Autodesk Inventor part; units mm, degrees
ref_plane "YZ Plane" through (0, 0, 0) normal (1, 0, 0) x (0, 1, 0)
ref_plane "XZ Plane" through (0, 0, 0) normal (0, 1, 0) x (-1, 0, 0)
ref_plane "XY Plane" through (0, 0, 0) normal (0, 0, 1) x (1, 0, 0)
sketch "Sketch1" plane through (0, 0, 0) normal (0, 1, 0) x (-1, 0, 0)
  line L0 (12.7, 14.875) -> (-12.7, 14.875)
  line L1 (-12.7, 14.875) -> (-12.7, -14.875)
  line L2 (-12.7, -14.875) -> (12.7, -14.875)
  line L3 (12.7, -14.875) -> (12.7, 14.875)
  point P0 (0, 0)
  dimension "d0" = 29.75
  dimension "d1" = 25.4
  dimension "d2" = 12.7
  dimension "d3" = 14.875
extrude "Extrusion1" add sketch "Sketch1" along normal blind 29.8
sketch "Sketch2" plane through (0, 29.8, 0) normal (0, 1, 0) x (1, 0, 0)
  circle A0 centre (0, 0) radius 5.35
  line L0 (12.7, 14.875) -> (-12.7, 14.875)
  line L1 (-12.7, 14.875) -> (-12.7, -14.875)
  line L2 (-12.7, -14.875) -> (12.7, -14.875)
  dimension "d7" = 10.7
  dimension "d8" = 14.875
  dimension "d9" = 12.7
  dimension "d12" = 14.875
extrude "Extrusion2" cut sketch "Sketch2" against normal through all
sketch "Sketch3" plane through (-12.7, 0, 14.875) normal (0, 0, 1) x (1, 0, 0)
  circle A0 centre (4.9, 24.9) radius 1.9
  circle A1 centre (21.4, 24.9) radius 1.9
  circle A2 centre (20.5, 4.9) radius 1.9
  circle A3 centre (4.9, 4.9) radius 1.9
  line L0 (0, 29.8) -> (25.4, 29.8)
  line L1 (0, 0) -> (0, 29.8)
  line L2 (0, 0) -> (25.4, 0)
  line L3 (25.4, 0) -> (25.4, 29.8)
  point P0 (12.7, 0)
  dimension "d13" = 3.8
  dimension "d14" = 3.8
  dimension "d15" = 3.8
  dimension "d16" = 3.8
  dimension "d17" = 4.9
  dimension "d18" = 4.9
  dimension "d19" = 4.9
  dimension "d20" = 4.9
  dimension "d21" = 4.9
  dimension "d22" = 4.9
  dimension "d23" = 4.9
  dimension "d24" = 4
hole "Hole1" at (-7.8, 24.9, 14.875) at (8.7, 24.9, 14.875) at (7.8, 4.9, 14.875) at (-7.8, 4.9, 14.875) direction (0, 0, -1) diameter 3.242 depth 11 tip angle 118 countersink diameter 4.3 countersink angle 90
sketch "Sketch4" plane through (0, 0, 0) normal (0, -1, 0) x (1, 0, 0)
  circle A0 centre (8, 0) radius 1.5
  circle A1 centre (0, -8) radius 1.5
  circle A2 centre (-8, 0) radius 1.5
  circle A3 centre (0, 8) radius 1.5
  line L0 (12.7, 14.875) -> (12.7, -14.875)
  line L1 (-12.7, -14.875) -> (-12.7, 14.875)
  line L2 (-12.7, 14.875) -> (12.7, 14.875)
  line L3 (12.7, -14.875) -> (-12.7, -14.875)
  point P0 (0, 0)
  dimension "d32" = 3
  dimension "d33" = 3
  dimension "d34" = 8
  dimension "d35" = 8
  dimension "d36" = 3
  dimension "d37" = 3
  dimension "d38" = 8
  dimension "d39" = 8
  dimension "d40" = 12.7
  dimension "d41" = 12.7
  dimension "d42" = 14.875
  dimension "d43" = 14.875
hole "Hole2" at (8, 0, 0) at (0, 0, -8) at (-8, 0, 0) at (0, 0, 8) direction (0, 1, 0) diameter 2.459 depth 10 tip angle 118 countersink diameter 3.01 countersink angle 90
properties part number "Z-AXIS SCREW SEAT"
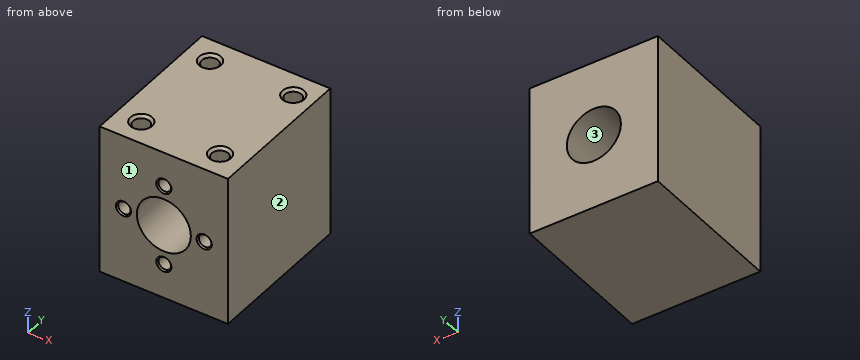
Input: part model. Units: mm. Frame: model coordinates. Face numbers are marked on the shaded views. Coordinates: 2 decimals unless noted, no trailing zeros. Loops run counter-clockwise (first coordinate to the right, second up) from the corner with the lowest first, then second, coordinate; pieces in that order, holes last.
Q1. Mould query, pull axis X, two halves, no side actions, for the marked faces 1, 2 and 3. Classes: +X half, -X half, draft (parallel to the pull), parting line (faces both ways), or undercut.
Results are:
face 1: draft
face 2: +X half
face 3: undercut
Q2. Section D-D, the plane y = 4.25. Give the number of separate pieces and of enclosed holes in the cut face, and give its area (3 significant figures).
Results are:
separate pieces: 1
enclosed holes: 5
area: 579 mm2
Q3. Section B-B, the plane y = 17. Return the cut outline in (x, z) (3 decimals), and give its area (3 significant figures).
Results are:
outline: (-12.7, -14.875) - (12.7, -14.875) - (12.7, 14.875) - (-12.7, 14.875) - close; hole circle Ø10.7 at (0, 0)
area: 666 mm2
Q4. Line query: line 1 along X through (y, z) = (24.9, 7.5); line 2 along X through (y, z) = (4.9, 6.5); line 3 along Z through (x, y) = (-8, 2.75) (1 decimal). Output: solid intervals per line, ascending.
Results are:
line 1: x = -12.7 to -9.42, -6.18 to 7.08, 10.32 to 12.7
line 2: x = -12.7 to -9.42, -6.18 to 6.18, 9.42 to 12.7
line 3: z = -14.9 to -1.2, 1.2 to 14.9
Q5. Section C-C, the plane x = -3. Return the cut outline in (y, z) (3 decimals).
Results are:
outline: (0, -14.875) - (29.8, -14.875) - (29.8, -4.43) - (0, -4.43) - close; (0, 4.43) - (29.8, 4.43) - (29.8, 14.875) - (0, 14.875) - close
Q6. Section A-A, the plane z = 11.5. Return the cut outline in (x, y).
Results are:
outline: (-12.7, 0) - (12.7, 0) - (12.7, 29.8) - (-12.7, 29.8) - close; hole circle Ø3.24 at (-7.8, 4.9); hole circle Ø3.24 at (-7.8, 24.9); hole circle Ø3.24 at (7.8, 4.9); hole circle Ø3.24 at (8.7, 24.9)
Q7. Contact query for flat-ended pins moving along their axis: pin 1 (3.5 mm diameter, centred on x = -7.8, y = 24.9, fed in from +Z) (3 decimals); pin 2 (2 mm diameter, centred on x = -8, z = 0, fed in from -Y); pin 3 (6.5 mm diameter, centred on x = 0, z = 0, fed in from +Y); pin 4 (4 mm diameter, centred on x = 7.8, y = 4.9, fed in from +Z) (3 decimals). Output: stop coordinate, or through.
Results are:
pin 1: stops at z = 14.475
pin 2: stops at y = 10.14
pin 3: passes through
pin 4: stops at z = 14.725
